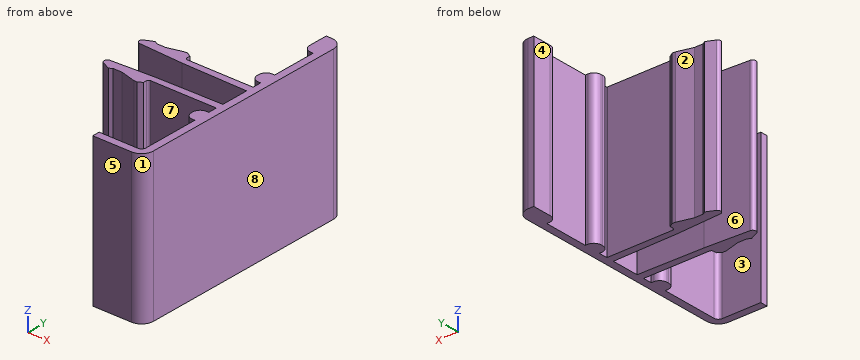
from build123d import *

# Parameters (mm, degrees)
MAIN_EXTRUSION_DEPTH = 25


with BuildPart() as part:
    # Sk Main Extrusion → Main Extrusion (new body)
    with BuildSketch(Plane.XY):
        with BuildLine():
            Line((-3.83, 2.5328), (-11.31249103, 2.925083334))
            ThreePointArc((-11.31249103, 2.925083334), (-11.819967595, 3.366238681), (-11.514691833, 3.965369062))
            Line((-11.514691833, 3.965369062), (-10.100108722, 4.625))
            Line((-10.100108722, 4.625), (-9.58, 4.3))
            Line((-9.58, 4.3), (-8.08, 4.3))
            Line((-8.08, 4.3), (-5.474147193, 5))
            Line((-5.474147193, 5), (-4.934147193, 5))
            Line((-4.934147193, 5), (-4.23, 4.56))
            Line((-4.23, 4.56), (-4.23, 4.025))
            ThreePointArc((-4.23, 4.025), (-4.112842712, 3.742157288), (-3.83, 3.625))
            Line((-3.83, 3.625), (7.27, 3.625))
            Line((7.27, 3.625), (7.27, 5.120055168))
            Line((7.27, 5.120055168), (6.79886836, 5.120055168))
            ThreePointArc((6.79886836, 5.120055168), (5.9740485, 5.504367154), (5.638, 6.35))
            Line((5.638, 6.35), (5.638, 6.65))
            ThreePointArc((5.638, 6.65), (5.9740485, 7.495632846), (6.79886836, 7.879944832))
            Line((6.79886836, 7.879944832), (7.27, 7.879944832))
            Line((7.27, 7.879944832), (7.27, 15.470020156))
            Line((7.27, 15.470020156), (6.798058361, 15.470020156))
            ThreePointArc((6.798058361, 15.470020156), (5.938401057, 15.86929153), (5.588, 16.75))
            Line((5.588, 16.75), (5.588, 20))
            Line((5.588, 20), (6.52, 20))
            ThreePointArc((6.52, 20), (7.934213562, 19.414213562), (8.52, 18))
            Line((8.52, 18), (8.52, -17.5))
            ThreePointArc((8.52, -17.5), (7.934213562, -18.914213562), (6.52, -19.5))
            Line((6.52, -19.5), (0, -19.5))
            Line((0, -19.5), (0, -18.25))
            Line((0, -18.25), (6.52, -18.25))
            ThreePointArc((6.52, -18.25), (7.050330086, -18.030330086), (7.27, -17.5))
            Line((7.27, -17.5), (7.27, -7.879944832))
            Line((7.27, -7.879944832), (6.79886836, -7.879944832))
            ThreePointArc((6.79886836, -7.879944832), (5.9740485, -7.495632846), (5.638, -6.65))
            Line((5.638, -6.65), (5.638, -6.35))
            ThreePointArc((5.638, -6.35), (5.9740485, -5.504367154), (6.79886836, -5.120055168))
            Line((6.79886836, -5.120055168), (7.27, -5.120055168))
            Line((7.27, -5.120055168), (7.27, -3.625))
            Line((7.27, -3.625), (-3.83, -3.625))
            ThreePointArc((-3.83, -3.625), (-4.112842712, -3.742157288), (-4.23, -4.025))
            Line((-4.23, -4.025), (-4.23, -4.56))
            Line((-4.23, -4.56), (-4.934147193, -5))
            Line((-4.934147193, -5), (-5.474147193, -5))
            Line((-5.474147193, -5), (-8.08, -4.3))
            Line((-8.08, -4.3), (-9.58, -4.3))
            Line((-9.58, -4.3), (-10.100108722, -4.625))
            Line((-10.100108722, -4.625), (-11.514691833, -3.965369062))
            ThreePointArc((-11.514691833, -3.965369062), (-11.819967595, -3.366238681), (-11.31249103, -2.925083334))
            Line((-11.31249103, -2.925083334), (-3.83, -2.5328))
            Line((-3.83, -2.5328), (7.27, -2.339048779))
            Line((7.27, -2.339048779), (7.27, 2.339048779))
            Line((7.27, 2.339048779), (-3.83, 2.5328))
        make_face()
    extrude(amount=-MAIN_EXTRUSION_DEPTH)


solid = part.part
The model under review builds one solid part; all positions refer to its coordinate system, in mm. Face numbers are marked on the shaded views. A direction names the side the tool comes from. Give positions to 0.01 mm unless a question says otherwise; leave off trailing zeros. Order: outer loops, then holes, each group sorted by start corner. A loop starts at its lowest first (then second) coordinate and runs counter-clockwise, first axis right, second up. Notation, with made-up numbers: M 26,-23 L 67,-23 A29 cw 67,9 Z; hole C 63,6 d7. An arc over 180 degrees is marked long. Answer in a Markdown table with one row per item. Add a question column.
1. Add section C-C on y = -9.5. State the section outline as (x, z) points, plus the area to 4 significant figures.
2. Add section A-A on x = -6.5. State the section outline as (y, z) points.
3. Add section B-B on x = 3. State the section outline as (y, z) points (3 decimals), plus the area to 3 significant figures.
4. Add section D-D on x = -9. State the section outline as (y, z) points, plus the area to 3 significant figures.
5. For pin 1 Ø1.5 at (x, z) = (-5.5, -4) entering from -Y; pin 2 Ø3.5 at (y, z) = (18.5, -7) entering from -X; pin 3 Ø10.5 at (y, z) = (-15, -18.5) entering from -X, all flat-tipped, find the tip position at first contact; note any pin that passes through.
6. Mouldability with a two-part tool opening along Y and no side actions: class the marked faces 1, 2 and 3 as released by +Y, released by -Y, zero draft, split by the parting line, or undercut.
7. Machinability: for the marked faces 4, 5, 6, 7 and 8, which of the approach directions +Z, -Z, +X, -X, +Y, -Y give a long, thin tool a straight path to every point of the face, cutting with its end or side? Answer none if there is none.
8. To check wall thickness, follow line 1 along Y through (x, z) = (6.75, -15) (3 decimals); line 2 along Y through (x, z) = (5.25, -21) (3 decimals); line 3 along X through (y, z) = (-14, -22). State the ranges of each line that lie inside material, in increasing order.
The answers:
| question | item | result |
|---|---|---|
| 1 | outline | M 7.27,-25 L 8.52,-25 L 8.52,0 L 7.27,0 Z |
| 1 | area | 31.25 mm2 |
| 2 | outline | M -4.72,-25 L -2.67,-25 L -2.67,0 L -4.72,0 Z; M 2.67,-25 L 4.72,-25 L 4.72,0 L 2.67,0 Z |
| 3 | outline | M -19.5,-25 L -18.25,-25 L -18.25,0 L -19.5,0 Z; M -3.625,-25 L -2.414,-25 L -2.414,0 L -3.625,0 Z; M 2.414,-25 L 3.625,-25 L 3.625,0 L 2.414,0 Z |
| 3 | area | 91.8 mm2 |
| 4 | outline | M -4.3,-25 L -2.8,-25 L -2.8,0 L -4.3,0 Z; M 2.8,-25 L 4.3,-25 L 4.3,0 L 2.8,0 Z |
| 4 | area | 74.8 mm2 |
| 5 | pin 1 | y = -5 |
| 5 | pin 2 | x = 5.59 |
| 5 | pin 3 | x = 0 |
| 6 | face 1 | released by -Y |
| 6 | face 2 | released by +Y |
| 6 | face 3 | undercut |
| 7 | face 4 | +Z, -Z, -X, +Y |
| 7 | face 5 | +Z, -Z, +X, -X, -Y |
| 7 | face 6 | +Z, -Z, -X |
| 7 | face 7 | +Z, -Z |
| 7 | face 8 | +Z, -Z, +X, +Y, -Y |
| 8 | line 1 | -19.487 to -18.214, -7.876 to -5.124, -3.625 to -2.348, 2.348 to 3.625, 5.124 to 7.876, 15.474 to 19.987 |
| 8 | line 2 | -19.5 to -18.25, -3.625 to -2.374, 2.374 to 3.625 |
| 8 | line 3 | 7.27 to 8.52 |
